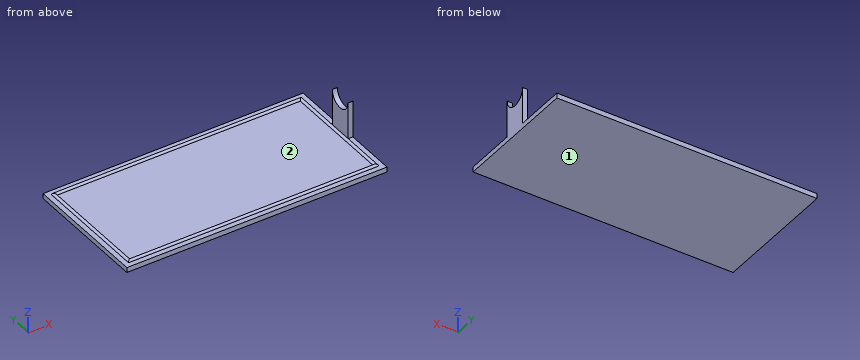
from build123d import *

# Parameters (mm, degrees)
ESQUISSE1_W             = 78
ESQUISSE1_H             = 38
BOSS_EXTRU_1_DEPTH      = 1.5
BALAYAGE1_PROFILE_R     = 0.5
ESQUISSE14_W            = 1.5
ESQUISSE14_H            = 7
BOSS_EXTRU_2_DEPTH      = 11
ENL_V_MAT_EXTRU_1_DEPTH = 11


with BuildPart() as part:
    # Esquisse1 → Boss.-Extru.1 (new body)
    with BuildSketch(Plane.XY):
        with Locations((39, 19)):
            Rectangle(ESQUISSE1_W, ESQUISSE1_H)
    extrude(amount=BOSS_EXTRU_1_DEPTH)

    # Balayage1: sweep along a curve in space
    with BuildLine() as balayage1_path:
        Line((2, 2, 1.5), (76, 2, 1.5))
        Line((76, 2, 1.5), (76, 36, 1.5))
        Line((76, 36, 1.5), (2, 36, 1.5))
        Line((2, 36, 1.5), (2, 2, 1.5))
    # Balayage1 profile (on start of the path) → Balayage1 (sweep)
    with BuildSketch(Plane(origin=(2, 2, 1.5), x_dir=(0, 0, 1), z_dir=(1, 0, 0))):
        Circle(BALAYAGE1_PROFILE_R)
    sweep(path=balayage1_path.line, transition=Transition.RIGHT)

    # Esquisse14 → Boss.-Extru.2 (add)
    with BuildSketch(Plane.XY.offset(1.5)):
        with Locations((77.25, 19)):
            Rectangle(ESQUISSE14_W, ESQUISSE14_H)
    extrude(amount=BOSS_EXTRU_2_DEPTH)

    # Esquisse15 → Enlèv. mat.-Extru.1 (cut)
    with BuildSketch(Plane(origin=(78, 0, 0), x_dir=(0, 0, -1), z_dir=(1, 0, 0))):
        with BuildLine():
            Line((-12.5, 15.5), (-14.376884621, 15.5))
            ThreePointArc((-14.376884621, 15.5), (-17.876884621, 19), (-14.376884621, 22.5))
            Line((-14.376884621, 22.5), (-12.5, 22.5))
            ThreePointArc((-12.5, 22.5), (-9, 19), (-12.5, 15.5))
        make_face()
    extrude(amount=-ENL_V_MAT_EXTRU_1_DEPTH, mode=Mode.SUBTRACT)


solid = part.part
Can you work these out from the model? Positions are in its coordinate system, mm. Face numbers are marked on the shaded views. Give positions to 0.01 mm unless a question says otherwise; leave off trailing zeros. Order: outer loops, then holes, each group sorted by start corner. A loop starts at its lowest first (then second) coordinate and runs counter-clockwise, first axis right, second up. Notation, with made-up numbers: M 89.5,48 L 121.5,48 A13 cw 121.5,61 Z; hole C 2,38 d3. An arc over 180 degrees is marked long. Use a Markdown table: item, result. Add a question column.
Item 1: Suppose I cut it at A-A (x = 34.5). List the corners of the cut face in (y, z) for me.
Item 2: We'd pull the mould along X, two halves only. Please class the marked faces 1 and 2: +X half, -X half, draft (parallel to the pull), parting line (faces both ways), or undercut.
Item 3: Suppose I cut it at B-B (y = 19). List the corners of the cut face in (x, z) for me, then the cut area to 3 significant figures.
Item 4: Will these pins go through, and if not, where does the flat tip stop? pin 1 (5 mm diameter, centred on x = 39, y = 10.5, fed in from +Z); pin 2 (1.6 mm diameter, centred on x = 77.5, z = 8.5, fed in from -Y); pin 3 (4 mm diameter, centred on y = 14, z = 5.5, fed in from -X).
Item 5: Suppose I cut it at C-C (z = 3.75). List the corners of the cut face in (x, y) for me.
Item 6: Suppose I cut it at D-D (y = 33). List the corners of the cut face in (x, z) for me.
Item 7: If I drill on L1, parallel to X at y = 21.5, z = 9.5; L2, parallel to Z at x = 32, y = 15, over which ranges is the centre line in solid material (lowest first)? Write a range as [from, to].
Answer sheet:
| question | item | result |
|---|---|---|
| 1 | outline | M 0,0 L 38,0 L 38,1.5 L 36.5,1.5 A0.5 ccw 35.5,1.5 L 2.5,1.5 A0.5 ccw 1.5,1.5 L 0,1.5 Z |
| 2 | face 1 | draft |
| 2 | face 2 | undercut |
| 3 | outline | M 0,0 L 78,0 L 78,9 L 76.5,9 L 76.5,1.5 A0.5 ccw 75.5,1.5 L 2.5,1.5 A0.5 ccw 1.5,1.5 L 0,1.5 Z |
| 3 | area | 129 mm² |
| 4 | pin 1 | stops at z = 1.5 |
| 4 | pin 2 | stops at y = 15.5 |
| 4 | pin 3 | stops at x = 76.5 |
| 5 | outline | M 76.5,15.5 L 78,15.5 L 78,22.5 L 76.5,22.5 Z |
| 6 | outline | M 0,0 L 78,0 L 78,1.5 L 76.5,1.5 A0.5 ccw 75.5,1.5 L 2.5,1.5 A0.5 ccw 1.5,1.5 L 0,1.5 Z |
| 7 | L1 | x = [76.5, 78] |
| 7 | L2 | z = [0, 1.5] |
